Could you check a few things on this model? Use its own coordinates, in mm. Face numbers are marked on the shaded views. A direction names the side the tool comes from. Give positions to 0.01 mm unless a question says otherwise; leave off trailing zeros. Order: outer loops, then holes, each group sorted by start corner. A loop starts at its lowest first (then second) coordinate and runs counter-clockwise, first axis right, second up. Notation, with made-up numbers: (29.5, -14) -> (79.5, -14) arc R17 cw to (79.5, 15) -> close; hole circle Ø1 at (59, -13.5). An arc over 180 degrees is marked (long way). Answer as CSV lines item,"result". Start each with the question number.
(1) I want a section at C-C (y = 49). Please give me the cut outline in (x, z).
(2) I need wall thicknesses on L1, parallel to Z at x = 46, y = 53; L2, parallel to Y at x = 15, z = 12; L3, parallel to Y at x = 13, z = 21.25. Which ranges of each line are inside material? Lowest first, please.
(3) On a 3-axis mill with a long thin cutter (end or side, diameter ignored), from which of +Z, -Z, +X, -X, +Y, -Y can I reach the whole of each face in a straight line? I mean the marked faces 1 and 2. Say none if no direction works.
(4) I want a section at A-A (y = 9.5). Please give me the cut outline in (x, z), plus the area to 3 significant figures.
(5) I want a section at B-B (x = 95). Please give me the cut outline in (y, z), plus the area to 3 significant figures.
(6) I want a section at D-D (x = 11.5). Please give me the cut outline in (y, z).
(7) Will these pins go through, and if not, where does the flat tip stop? pin 1 Ø6 at (x, y) = (77, 30.5) entering from +Z; pin 2 Ø1 at (x, y) = (63.5, 28) entering from -Z; pin 3 Ø1 at (x, z) = (67.5, 5) entering from +Y.
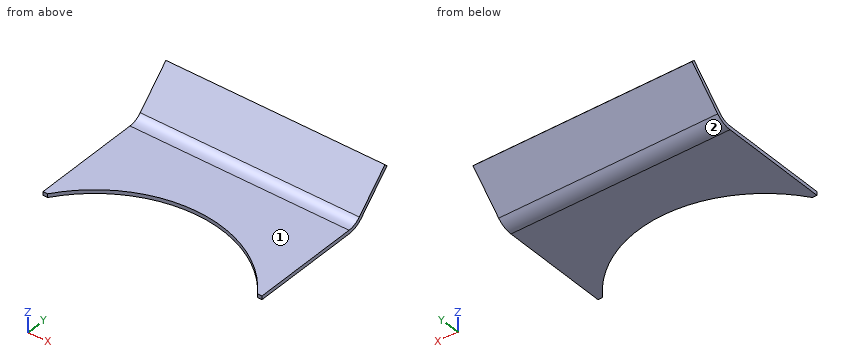
```python
from build123d import *

# Parameters (mm, degrees)
SKETCH_2_W             = 120
SKETCH_2_H             = 60
SM_BASE_FLANGE_1_DEPTH = 2
SM_EDGE_FLANGE_1_DEPTH = 120
CUT_EXTRUDE_3_REACH    = 151.465
SKETCH_3_R             = 70


# Sheet-metal steps are written as plain solids
with BuildPart() as part:
    # Sketch 2 → Базовая кромка1 (new body)
    with BuildSketch(Plane.XY):
        with Locations((60, 30)):
            Rectangle(SKETCH_2_W, SKETCH_2_H)
    extrude(amount=SM_BASE_FLANGE_1_DEPTH)

    # Ребро-кромка1 section (across the edge) → Ребро-кромка1 (add)
    with BuildSketch(Plane(origin=(120, 64.142135624, 2), x_dir=(0, -0.7071067811865438, 0.7071067811865512), z_dir=(-1, 0, 0))):
        with BuildLine():
            Line((-2, 4.142135624), (-2, 29.171572875))
            Line((-2, 29.171572875), (0, 29.171572875))
            Line((0, 29.171572875), (0, 4.142135624))
            ThreePointArc((0, 4.142135624), (0.761204675, 0.3153013), (2.928932188, -2.928932188))
            Line((2.928932188, -2.928932188), (1.514718626, -4.343145751))
            ThreePointArc((1.514718626, -4.343145751), (-1.08655439, -0.450065565), (-2, 4.142135624))
        make_face()
    extrude(amount=SM_EDGE_FLANGE_1_DEPTH)

    # Эскиз3 → Вырез-Вытянуть3 (cut, up to next)
    with BuildSketch(Plane.XY, mode=Mode.PRIVATE) as cut_extrude_3_sk1:
        with Locations((60, -40)):
            Circle(SKETCH_3_R)
    cut_extrude_3_tool1 = extrude(cut_extrude_3_sk1.sketch, amount=CUT_EXTRUDE_3_REACH, mode=Mode.PRIVATE) & part.part
    add(cut_extrude_3_tool1.solids().sort_by_distance((60, -40, 0))[0], mode=Mode.SUBTRACT)


solid = part.part
```
Final values:
1,outline,"(0, 0) -> (120, 0) -> (120, 2) -> (0, 2) -> close"
2,L1,"0 to 2"
2,L2,"74.14 to 76.97"
2,L3,"83.39 to 86.15"
3,face 1,"+Z, +X, -X, -Y"
3,face 2,"-Z, +X, -X, +Y"
4,outline,"(0, 0) -> (10.51, 0) -> (10.51, 2) -> (0, 2) -> close; (109.49, 0) -> (120, 0) -> (120, 2) -> (109.49, 2) -> close"
4,area,"42.0 mm²"
5,outline,"(20.62, 0) -> (60, 0) arc R12 ccw to (68.49, 3.51) -> (86.18, 21.21) -> (84.77, 22.63) -> (67.07, 4.93) arc R10 cw to (60, 2) -> (20.62, 2) -> close"
5,area,"146 mm²"
6,outline,"(10.48, 0) -> (60, 0) arc R12 ccw to (68.49, 3.51) -> (86.18, 21.21) -> (84.77, 22.63) -> (67.07, 4.93) arc R10 cw to (60, 2) -> (10.48, 2) -> close"
7,pin 1,"z = 2"
7,pin 2,"through"
7,pin 3,"y = 70.47"
